Can you work these out from the drawing? Everything is in mm from the part's minimum corner. Coordinates: 2 decimals unless noted, no trailing zeros. Order: outer loops, then holes, each group sorted by start corner. A loop starts at its lowest first (then second) coordinate and runs counter-clockwise, first axis right, second up. Notation, with made-up numbers: (54, 65) - (68, 65) arc R3 ccw to (68, 70) - close; hole circle Ø11 at (75.25, 26). An arc over 180 degrees is marked (long way). Answer as CSV lines item,"result". Start each with the question number.
Q1. Suppose I cut it at D-D (y = 33.8). Please give me the cut outline in (x, z).
Q2. Suppose I cut it at C-C (z = 0.35). Please give me the cut outline in (x, y).
Q3. For pin 1 Ø1 at (y, z) = (11, 1.5) entering from +X; pin 2 Ø0.6 at (x, z) = (35, 1.5) entering from -Y; pin 3 Ø0.6 at (y, z) = (8, 1) entering from -X, each with a flat end and sliding along its axis, tell me the tip position at first contact or that it passes through.
Q4. Suppose I cut it at B-B (y = 7.5). Please give me the cut outline in (x, z).
Q5. I need wall thicknesses on line 1 (Y direction, x = 42, z = 1); line 2 (X direction, y = 15, z = 0.45); line 3 (X direction, y = 50.5, z = 1.6) (1 decimal). Which ranges of each line are inside material? Lowest first, please.
Q6. Suppose I cut it at A-A (x = 39.5). Please give me the cut outline in (y, z).
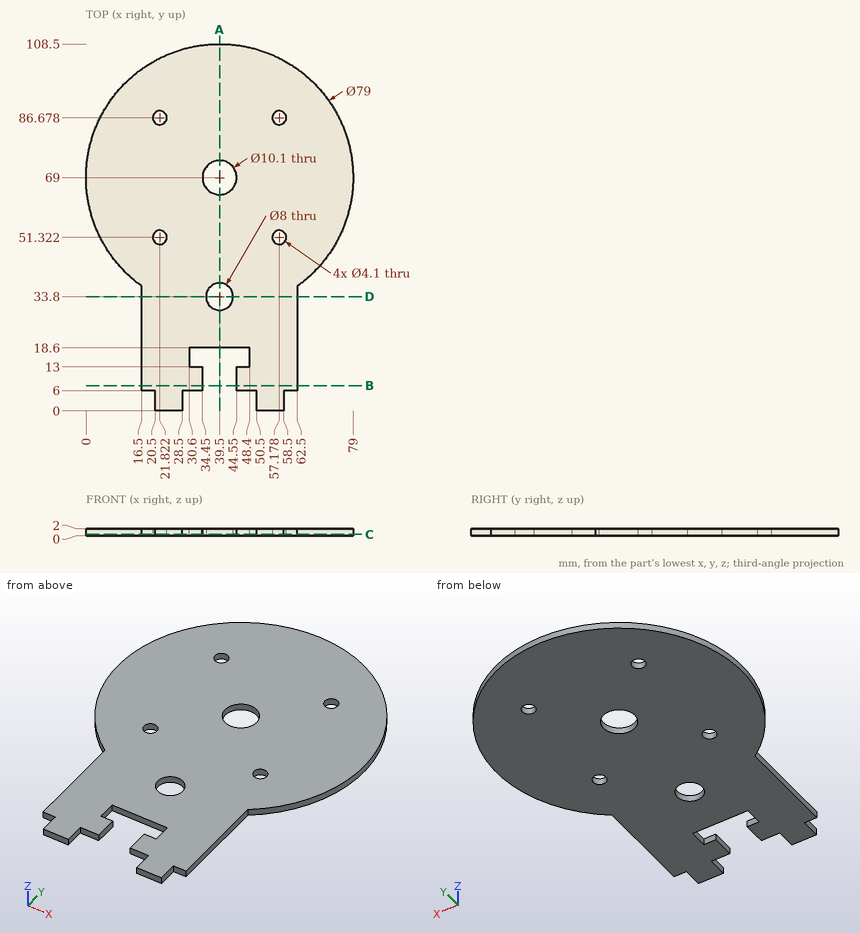
Here are the results:
1,outline,"(16.5, 0) - (35.5, 0) - (35.5, 2) - (16.5, 2) - close; (43.5, 0) - (62.5, 0) - (62.5, 2) - (43.5, 2) - close"
2,outline,"(16.5, 6) - (20.5, 6) - (20.5, 0) - (28.5, 0) - (28.5, 6) - (34.45, 6) - (34.45, 13) - (30.6, 13) - (30.6, 18.6) - (48.4, 18.6) - (48.4, 13) - (44.55, 13) - (44.55, 6) - (50.5, 6) - (50.5, 0) - (58.5, 0) - (58.5, 6) - (62.5, 6) - (62.5, 36.89) arc R39.5 ccw (long way) to (16.5, 36.89) - close; hole circle Ø4.1 at (21.82, 51.32); hole circle Ø4.1 at (21.82, 86.68); hole circle Ø10.1 at (39.5, 69); hole circle Ø8 at (39.5, 33.8); hole circle Ø4.1 at (57.18, 51.32); hole circle Ø4.1 at (57.18, 86.68)"
3,pin 1,"stops at x = 62.5"
3,pin 2,"stops at y = 18.6"
3,pin 3,"stops at x = 16.5"
4,outline,"(16.5, 0) - (34.45, 0) - (34.45, 2) - (16.5, 2) - close; (44.55, 0) - (62.5, 0) - (62.5, 2) - (44.55, 2) - close"
5,line 1,"y = 18.6 to 30.68, 36.92 to 64.61, 73.39 to 108.42"
5,line 2,"x = 16.5 to 30.6, 48.4 to 62.5"
5,line 3,"x = 4.6 to 19.9, 23.7 to 55.3, 59.1 to 74.4"
6,outline,"(18.6, 0) - (29.8, 0) - (29.8, 2) - (18.6, 2) - close; (37.8, 0) - (63.95, 0) - (63.95, 2) - (37.8, 2) - close; (74.05, 0) - (108.5, 0) - (108.5, 2) - (74.05, 2) - close"
